Design review of the part built by this model. Coordinates are the model's own, in mm. A direction names the side the tool comes from. Round coordinates to 2 decimals unless told otherwise and drop trailing zeros. Order: outer loops, then holes, each group sorted by start corner. A loop starts at its lowest first (then second) coordinate and runs counter-clockwise, first axis right, second up. Notation, with made-up numbers: M 74,25.25 L 81,25.25 A33 ccw 81,54.25 Z; hole C 87.5,21.25 d5. An arc over 180 degrees is marked long. Write each question's results on one line, items separated by ' | '. Start each with the question number.
Item 1: Machinability: for faces 1 (the flat face through (14.5, 0, -17)), 2 (the flat face through (-2, -4, -19)), 3 (the flat face through (3, 3, -18)), 4 (the flat face through (-24, 0, -5)), which of the approach directions +Z, -Z, +X, -X, +Y, -Y give a long, thin tool a straight path to every point of the face, cutting with its end or side? Answer none if there is none.
Item 2: Take a section at B-B, the plane x = 0. Write out the cut boundary in (y, z).
Item 3: Wall thickness on line 1 (X direction, y = -4.7, z = -15); line 2 (X direction, y = 2.5, z = -20.5); line 3 (X direction, y = 4.6, z = -15): over which ranges is each line inside the solid? List them lowest first. Write a range as [from, to].
Item 4: Take a section at D-D, the plane x = 20.5. Write out the cut boundary in (y, z).
Item 5: Take a section at C-C, the plane y = 4. Write out the cut boundary in (x, z), plus the area to 3 significant figures.
Item 6: Clearance check with flat-ended pins moving along their axes: pin 1 (6.5 mm diameter, centred on x = 20.5, y = 0, fed in from -Z); pin 2 (2 mm diameter, centred on y = -4, z = -24.5, fed in from -X); pin 3 (20 mm diameter, centred on x = 0, z = -15, fed in from -Y); pin 4 (14.5 mm diameter, centred on x = 0, z = -15, fed in from -Y). State where each tip first meets the part, or that it passes through.
Item 7: The part is to be moulded in two halves that separate along Y. For faces 5 (the flat face through (0, 6, -1)), 6 (the cylindrical face through (-2.4, -0.5, -18.2)), 7 (the cylindrical face through (-17.753, 0.121, -0.07)), 8 (the cylindrical face through (23.247, 0.121, -0.07)), say which applies: +Y half, -Y half, draft (parallel to the pull), parting line (faces both ways), or undercut.
Item 8: Take a section at A-A, the plane y = 0. Write out the cut boundary in (x, z), plus the area to 3 significant figures.
```python
from build123d import *

# Parameters (mm, degrees)
EXTRUDE_1_DEPTH     = 6
FILLET_1_R          = 2
SKETCH_2_R          = 2.75
CUT_EXTRUDE_1_DEPTH = 140
SKETCH_3_R          = 9
CUT_EXTRUDE_2_DEPTH = 2
SKETCH_5_R          = 12.5
CUT_EXTRUDE_4_DEPTH = 3
SKETCH_6_R          = 4
CUT_EXTRUDE_5_DEPTH = 76


with BuildPart() as part:
    # 草图1 → 凸台-拉伸1 (new, symmetric)
    with BuildSketch(Plane(origin=(0, 0, 0), x_dir=(1, 0, 0), z_dir=(0, 1, 0))):
        with BuildLine():
            Line((14.5, 5), (26.5, 5))
            Line((26.5, 5), (26.5, -5))
            Line((26.5, -5), (-26.5, -5))
            Line((-26.5, -5), (-26.5, 5))
            Line((-26.5, 5), (-14.5, 5))
            Line((-14.5, 5), (-14.5, 27))
            ThreePointArc((-14.5, 27), (-13.035533906, 30.535533906), (-9.5, 32))
            Line((-9.5, 32), (9.5, 32))
            ThreePointArc((9.5, 32), (13.035533906, 30.535533906), (14.5, 27))
            Line((14.5, 27), (14.5, 5))
        make_face()
    extrude(amount=EXTRUDE_1_DEPTH, both=True)

    # 圆角1
    fillet_1_edges = [part.edges().sort_by_distance(p)[0] for p in [
        (-14.5, 0, -5),
        (14.5, 0, -5),
    ]]
    fillet(fillet_1_edges, radius=FILLET_1_R)

    # 草图2 → 切除-拉伸1 (cut, symmetric)
    with BuildSketch(Plane(origin=(0, 0, -5), x_dir=(-1, 0, 0), z_dir=(0, 0, -1))):
        with Locations((20.5, 0)):
            Circle(SKETCH_2_R)
        with Locations((-20.5, 0)):
            Circle(SKETCH_2_R)
    extrude(amount=CUT_EXTRUDE_1_DEPTH, both=True, mode=Mode.SUBTRACT)

    # 草图3 → 切除-拉伸2 (cut)
    with BuildSketch(Plane.XZ.offset(6)):
        with Locations(Location((0, -15, 0), (0, 0, 270))):
            Circle(SKETCH_3_R)
    extrude(amount=-CUT_EXTRUDE_2_DEPTH, mode=Mode.SUBTRACT)

    # 草图5 → 切除-拉伸4 (cut)
    with BuildSketch(Plane(origin=(0, 6, 0), x_dir=(1, 0, 0), z_dir=(0, 1, 0))):
        with Locations(Location((0, 15, 0), (0, 0, 270))):
            Circle(SKETCH_5_R)
    extrude(amount=-CUT_EXTRUDE_4_DEPTH, mode=Mode.SUBTRACT)

    # 草图6 → 切除-拉伸5 (cut)
    with BuildSketch(Plane(origin=(0, 3, 0), x_dir=(1, 0, 0), z_dir=(0, 1, 0))):
        with Locations(Location((0, 15, 0), (0, 0, 270))):
            Circle(SKETCH_6_R)
    extrude(amount=-CUT_EXTRUDE_5_DEPTH, mode=Mode.SUBTRACT)


solid = part.part
```
Results list:
1) face 1: -Z, +X, +Y, -Y | face 2: -Y | face 3: +Y | face 4: -Z, -X, +Y, -Y
2) outline: M -6,-32 L 6,-32 L 6,-27.5 L 3,-27.5 L 3,-19 L -4,-19 L -4,-24 L -6,-24 Z; M -6,-6 L -4,-6 L -4,-11 L 3,-11 L 3,-2.5 L 6,-2.5 L 6,5 L -6,5 Z
3) line 1: [-14.5, -9], [9, 14.5] | line 2: [-14.5, 14.5] | line 3: [-14.5, -12.5], [12.5, 14.5]
4) outline: M -6,-5 L -2.75,-5 L -2.75,5 L -6,5 Z; M 2.75,-5 L 6,-5 L 6,5 L 2.75,5 Z
5) outline: M -26.5,-5 L -16.5,-5 A2 cw -14.5,-7 L -14.5,-27 A5 ccw -9.5,-32 L 9.5,-32 A5 ccw 14.5,-27 L 14.5,-7 A2 cw 16.5,-5 L 26.5,-5 L 26.5,5 L -26.5,5 Z; hole C 0,-15 d25 | area: 813 mm²
6) pin 1: z = -5 | pin 2: x = -14.5 | pin 3: y = -6 | pin 4: y = -4
7) face 5: +Y half | face 6: draft | face 7: undercut | face 8: undercut
8) outline: M -26.5,-5 L -23.25,-5 L -23.25,5 L -26.5,5 Z; M -17.75,-5 L -16.5,-5 A2 cw -14.5,-7 L -14.5,-27 A5 ccw -9.5,-32 L 9.5,-32 A5 ccw 14.5,-27 L 14.5,-7 A2 cw 16.5,-5 L 17.75,-5 L 17.75,5 L -17.75,5 Z; M 23.25,-5 L 26.5,-5 L 26.5,5 L 23.25,5 Z; hole C 0,-15 d8 | area: 1,140 mm²
